Geometry: final body of the model. Coordinates: model frame, mm. A direction names the side the tool comes from. Give positions to 0.01 mm unless a question says otherwise; leave off trailing zeros. Write each loop counter-clockwise with the first axis right and the second up, starting at its lowest first coordinate (ties: lowest second). Pieces come first, ordered by that corner, then holes.
from build123d import *

# Parameters (mm, degrees)
SKETCH1_W      = 5
SKETCH1_H      = 22
SKETCH2_R      = 11
EXTRUDE1_DEPTH = 25
HOLEWZD1_D     = 5.4
HOLEWZD2_D     = 10
HOLEWZD2_DEPTH = 30
CHAMFER1_SIZE  = 0.5
CHAMFER2_SIZE  = 1
FILLET1_R      = 0.4


with BuildPart() as part:
    # Sketch1 → Revolve1 (revolve)
    with BuildSketch(Plane(origin=(0, 0, 0), x_dir=(-1, 0, 0), z_dir=(0, 0, -1))):
        with Locations((-2.5, 11)):
            Rectangle(SKETCH1_W, SKETCH1_H)
    revolve(axis=Axis((5, 0, 0), (-1, 0, 0)))

    # Sketch2 → Extrude1 (add)
    with BuildSketch(Plane(origin=(5, 0, 0), x_dir=(0, 0, -1), z_dir=(1, 0, 0))):
        Circle(SKETCH2_R)
    extrude(amount=EXTRUDE1_DEPTH)

    # HoleWzd1 (through all)
    with Locations(Plane(origin=(5, 0, 0), x_dir=(0, 0, -1), z_dir=(1, 0, 0))):
        with Locations((0, -15.5), (15.5, 0), (-15.5, 0), (0, 15.5)):
            Hole(HOLEWZD1_D / 2)

    # HoleWzd2
    with Locations(Plane(origin=(30, 0, 0), x_dir=(0, 0, -1), z_dir=(1, 0, 0))):
        with Locations((0, 0)):
            Hole(HOLEWZD2_D / 2, depth=HOLEWZD2_DEPTH)

    # Chamfer1
    chamfer1_edges = [part.edges().sort_by_distance(p)[0] for p in [
        (0, -22, 0),
        (5, -22, 0),
        (30, 0, 11),
    ]]
    chamfer(chamfer1_edges, length=CHAMFER1_SIZE)

    # Chamfer2
    chamfer2_edges = [part.edges().sort_by_distance(p)[0] for p in [
        (30, 0, -5),
        (0, 0, -5),
    ]]
    chamfer(chamfer2_edges, length=CHAMFER2_SIZE)

    # Fillet1
    fillet1_edges = [part.edges().sort_by_distance(p)[0] for p in [
        (5, 0, 11),
    ]]
    fillet(fillet1_edges, radius=FILLET1_R)


solid = part.part
Q1. Pin query (flat end, axial travel): P1, Ø2, axis at x = 17, z = -5, coming from the +Y side; P2, Ø3, axis at y = -15.5, z = 0, coming from the -X side (1 decimal); P3, Ø8, axis at x = 18.5, z = 8.5, coming from the +Y side; P4, Ø1, axis at x = 9, y = -7, coming from the -Z side. Return the tip coordinate at first contact, or that it passes through.
Filled sheet:
P1: stops at y = 10.25
P2: passes through
P3: stops at y = 10.04
P4: stops at z = -8.87
Q2. Pull-direction query (Z, two-part tool) for faces 1 (the cylindrical face through (2.472, -4.769, 21.477)), 2 (the flat face through (30, -5, -5)), 3 (the cylindrical face through (14.8, -4.88, -1.08)); classes: released by +Z, released by -Z, zero draft, split by the parting line, or undercut.
Filled sheet:
face 1: split by the parting line
face 2: zero draft
face 3: undercut
Q3. Section C-C on x = 11.25. Output: boundary loops of the cut face in (y, z).
Filled sheet:
outline: circle Ø22 at (0, 0); hole circle Ø10 at (0, 0)
Q4. Ray query, line 1 along Y through (x, z) = (24, 4.5); line 2 along Y through (x, z) = (13.75, -3.5); line 3 along Y through (x, z) = (4.75, -1). Return the intervals inside material, ascending.
Filled sheet:
line 1: y = -10.04 to -2.18, 2.18 to 10.04
line 2: y = -10.43 to -3.57, 3.57 to 10.43
line 3: y = -21.73 to -18.01, -12.99 to -4.9, 4.9 to 12.99, 18.01 to 21.73
Q5. Access query for faces 4 (the cylindrical face through (17.28, -10.74, 2.38)), 5 (the cylindrical face through (2.465, 18.177, -0.351)). Directions: +Z, -Z, +X, -X, +Y, -Y. A direction counts if a zero-diameter tool reaches every point of the face in a straight line with its end or side. Return the directions, or none.
Filled sheet:
face 4: +X
face 5: +X, -X
Q6. Section A-A on z = 0. Count the separate pieces of the cut face and the enclosed holes in it, plus the area to 3 significant figures.
Filled sheet:
separate pieces: 4
enclosed holes: 0
area: 413 mm2
